Autodesk Inventor part; units mm, degrees
ref_plane "YZ Plane" through (0, 0, 0) normal (1, 0, 0) x (0, 1, 0)
ref_plane "XZ Plane" through (0, 0, 0) normal (0, 1, 0) x (-1, 0, 0)
ref_plane "XY Plane" through (0, 0, 0) normal (0, 0, 1) x (1, 0, 0)
sketch "Sketch1" plane through (0, 0, 0) normal (1, 0, 0) x (0, 1, 0)
  line L0 (0, 0) -> (0, 25.4)
  line L1 (3.175, 28.575) -> (28.575, 28.575)
  line L2 (31.75, 25.4) -> (31.75, 0)
  line L3 (28.575, 0) -> (28.575, 25.4)
  line L4 (28.575, 25.4) -> (3.175, 25.4)
  line L5 (3.175, 25.4) -> (3.175, 0)
  line L6 (0, 0) -> (3.175, 0)
  line L7 (28.575, 0) -> (31.75, 0)
  arc A0 (3.175, 28.575) -> (0, 25.4) centre (3.175, 25.4) ccw
  arc A1 (31.75, 25.4) -> (28.575, 28.575) centre (28.575, 25.4) ccw
  point P0 (0, 28.575)
  point P1 (31.75, 28.575)
  dimension "d0" = 28.575
  dimension "d2" = 31.75
  dimension "d3" = 90
  dimension "d4" = 28.575
  dimension "d5" = 90
  dimension "d6" = 3.175
  dimension "d7" = 3.175
extrude "Extrusion1" add sketch "Sketch1" along normal blind 406.4
sketch "Sketch2" plane through (0, 31.75, 25.4) normal (0, 1, 0) x (1, 0, 0)
  line L0 (0, 0) -> (0, 25.4)
  line L1 (0, 0) -> (406.4, 0)
  line L2 (406.4, 25.4) -> (406.4, 0)
  line L3 (0, 25.4) -> (406.4, 25.4)
  point P0 (0, 25.4)
  point P1 (12.7, 12.7)
  dimension "d10" = 12.7
  dimension "d11" = 12.7
hole "Hole1" at (12.7, 31.75, 12.7) direction (0, -1, 0) diameter 6.35 end through all
pattern_linear "Rectangular Pattern1" count 20 spacing 25.4 along (1, 0, 0) of "Hole1"
sketch "Sketch4" plane through (0, 3.175, 28.575) normal (0, 0, 1) x (1, 0, 0)
  line L0 (0, 0) -> (0, 25.4)
  line L1 (0, -3.175) -> (0, 0)
  line L2 (0, -3.175) -> (406.4, -3.175)
  line L3 (406.4, 0) -> (406.4, -3.175)
  line L4 (0, 0) -> (406.4, 0)
  point P0 (0, -3.175)
  point P1 (15.875, 14.2875)
  point P2 (139.7, 14.2875)
  dimension "d28" = 15.875
  dimension "d30" = 139.7
  dimension "d45" = 17.4625
  dimension "d46" = 17.4625
hole "Hole2" at (15.875, 17.4625, 28.575) at (139.7, 17.4625, 28.575) direction (0, 0, -1) diameter 6.35 end through all
sketch "Sketch5" plane through (0, 0, 0) normal (-1, 0, 0) x (0, 0, 1)
  line L0 (0, 0) -> (25.4, 0)
  arc A0 (25.4, 0) -> (28.575, 3.175) centre (25.4, 3.175) ccw
  line L1 (28.575, 3.175) -> (28.575, 28.575)
  arc A1 (28.575, 28.575) -> (25.4, 31.75) centre (25.4, 28.575) ccw
  line L2 (25.4, 31.75) -> (0, 31.75)
  line L3 (0, 31.75) -> (0, 28.575)
  line L4 (0, 28.575) -> (25.4, 28.575)
  line L5 (25.4, 28.575) -> (25.4, 3.175)
  line L6 (25.4, 3.175) -> (0, 3.175)
  line L7 (0, 3.175) -> (0, 0)
  line L8 (0, 0) -> (25.4, 0)
  line L9 (25.4, 0) -> (25.4, 3.175)
extrude "Extrusion3" add sketch "Sketch5" along normal blind 25.4 contours L9 L5 L4 L3 L2 A1 L1 A0
sketch "Sketch6" plane through (406.4, 31.75, 25.4) normal (0, 1, 0) x (1, 0, 0)
  line L0 (0, 25.4) -> (-431.8, 25.4)
  line L1 (-431.8, 0) -> (-431.8, 25.4)
  circle A0 centre (-419.1, 12.7) radius 3.175
  point P0 (-406.4, 25.4)
  dimension "d40" = 6.35
  dimension "d41" = 12.7
  dimension "d42" = 12.7
extrude "Extrusion4" cut sketch "Sketch6" against normal blind 25.4
fillet "Fillet1" radius 3.175 2 edges at (203.2, 3.175, 25.4) (190.5, 28.575, 25.4)
properties part number "c-channel"
Can you work these out from the model? Positions are in its coordinate system, mm. A direction names the side the tool comes from. Round coordinates to 2 decimals unless told otherwise and drop trailing zeros. Order: outer loops, then holes, each group sorted by start corner. A loop starts at its lowest first (then second) coordinate and runs counter-clockwise, first axis right, second up. Notation, with made-up numbers: M -10.75,-27.5 L 8.25,-27.5 A5 cw 8.25,-18.5 Z; hole C 16,-16.5 d7. An arc over 180 degrees is marked long. Use a Markdown table: item, result.
1) I'm going to push flat-ended pins straight in: P1, Ø10, axis at y = 19, z = 18, coming from the +X side; P2, Ø12.5, axis at x = 123.5, y = 15, coming from the -Z side; P3, Ø1.5, axis at y = 3.5, z = 13, coming from the -X side. Where does each tip first touch, or does it pass through?
Geometry says:
| item | result |
|---|---|
| P1 | passes through |
| P2 | stops at z = 25.4 |
| P3 | stops at x = 0 |
2) Imagine slicing it at A-A (x = 330.5). List the corners of the cut face in (y, z) for me (3 decimals).
Geometry says:
| item | result |
|---|---|
| outline | M 0,0 L 3.175,0 L 3.175,22.225 A3.175 cw 6.35,25.4 L 25.4,25.4 A3.175 cw 28.575,22.225 L 28.575,0 L 31.75,0 L 31.75,25.4 A3.175 ccw 28.575,28.575 L 3.175,28.575 A3.175 ccw 0,25.4 Z |
3) On a 3-axis mill with a long thin cutter (end or side, diameter ignored), from which of +Z, -Z, +X, -X, +Y, -Y can I reach the whole of each face in a straight line? I mean faces 4 (the face through (194, 31.75, 10)), 5 (the face through (194, 28.575, 11)). Say none if no direction works.
Geometry says:
| item | result |
|---|---|
| face 4 | +Z, -Z, +X, -X, +Y |
| face 5 | -Z, +X, -X |
4) If I drill on line 1 along Y through (x, z) = (150, 11.5) (3 decimals); line 2 along Z through (x, y) = (256.5, 8) (3 decimals); line 3 along Z through (x, y) = (139.7, 1.35) (3 decimals), over which ranges is the centre line in solid material (lowest first)?
Geometry says:
| item | result |
|---|---|
| line 1 | y = 0 to 3.175, 28.575 to 31.75 |
| line 2 | z = 25.4 to 28.575 |
| line 3 | z = 0 to 9.525, 15.875 to 27.998 |
5) If we mould it in two halves opening along Y, with no side actions, what happens to faces 1 (the face through (194, 15, 25.4)), 2 (the face through (194, 16, 28.575)), 3 (the face through (200, 0, 13))? For each: +Y half, -Y half, draft (parallel to the pull), parting line (faces both ways), or undercut.
Geometry says:
| item | result |
|---|---|
| face 1 | undercut |
| face 2 | draft |
| face 3 | -Y half |
